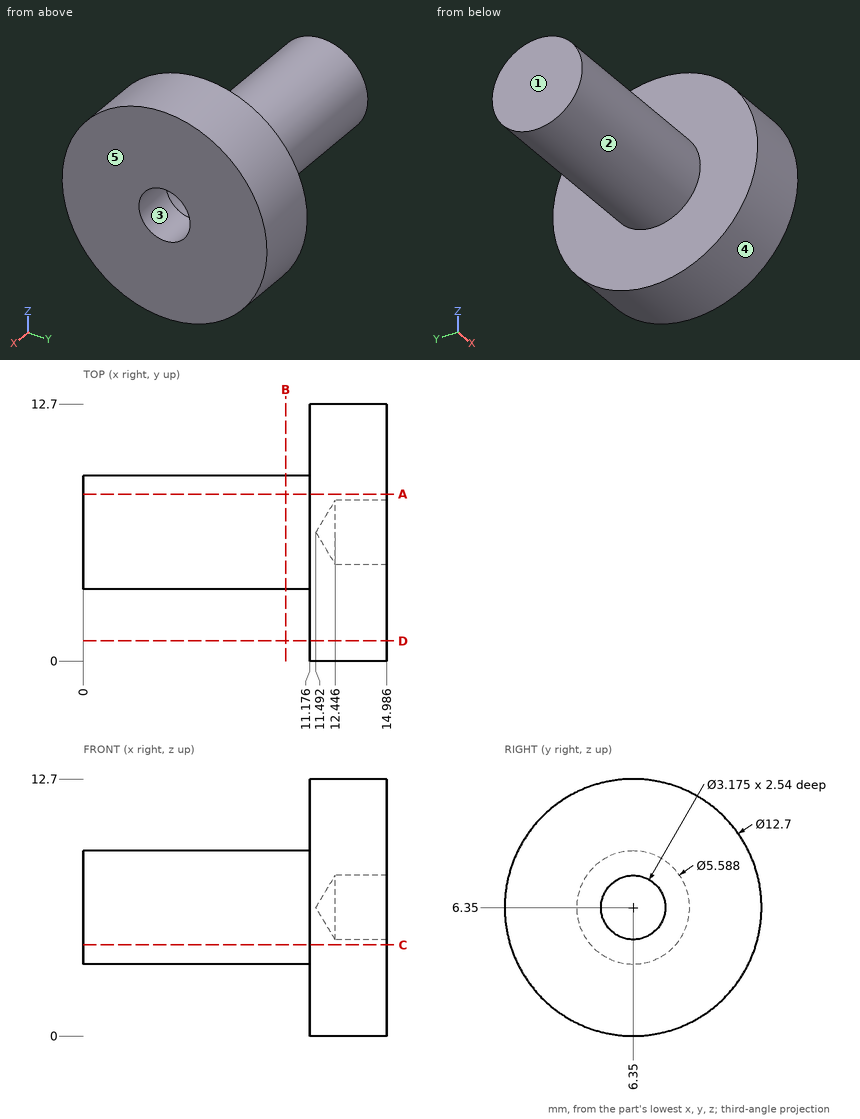
Answer from the drawing. Dimensions are ordinates in mm from the lowest x, y and z of the part. A direction names the side the tool comes from. Give positions to 0.01 mm unless a question says otherwise; leave off trailing zeros. Write each loop counter-clockwise with the first axis right and the second up, starting at its lowest first coordinate (ties: lowest second). Pieces come first, ordered by that corner, then holes.
1) Section C-C (z = 4.5) is taken. Write down the section's boundary in (x, y).
2) A tool of negligible diameter and unlimited length cuts with its end or side. For the marked faces 1 and 2, from which of +Z, -Z, +X, -X, +Y, -Y can it reach the whole face along a straight path? Write none if from no direction.
3) Section D-D (y = 1) is taken. Write down the section's boundary in (x, z), and give its area (3 significant figures).
4) Given P1, Ø6, axis at x = 1.5, y = 11, coming from the -Z side (1 decimal); P2, Ø1, axis at x = 7, z = 4.5, coming from the -Y side; P3, Ø1, axis at x = 4, z = 9, coming from the -Y side (1 decimal), each flat-ended and moving along its own axis, determine where each tip first touches the part or whether it passes through.
5) Find the intervals of material crossed by L1, parallel to Y at x = 14.1, z = 6.35; L2, parallel to X at y = 8.25, z = 10.75; L3, parallel to Z at x = 4.25, y = 6.5, in increasing order.
6) For a pull along Y with two mould halves and no side action, classify the marked faces 3, 4 and 5 as pulls with the +Y half, pulls with the -Y half, needs draft (parallel to the pull), parting line crosses it, or undercut.
7) Section B-B (x = 10) is taken. Write down the section's boundary in (y, z), and give its area (3 significant figures).
8) Section A-A (y = 8.25) is taken. Write down the section's boundary in (x, z).
Response:
1. outline: (0, 4.26) - (11.18, 4.26) - (11.18, 0.28) - (14.99, 0.28) - (14.99, 12.42) - (11.18, 12.42) - (11.18, 8.44) - (0, 8.44) - close
2. face 1: +Z, -Z, -X, +Y, -Y
2. face 2: -X
3. outline: (11.18, 2.93) - (14.99, 2.93) - (14.99, 9.77) - (11.18, 9.77) - close
3. area: 26.1 mm2
4. P1: stops at z = 4.1
4. P2: stops at y = 3.9
4. P3: stops at y = 4.6
5. L1: y = 0 to 4.76, 7.94 to 12.7
5. L2: x = 11.18 to 14.99
5. L3: z = 3.56 to 9.14
6. face 3: undercut
6. face 4: parting line crosses it
6. face 5: needs draft
7. outline: circle Ø5.59 at (6.35, 6.35)
7. area: 24.5 mm2
8. outline: (0, 4.3) - (11.18, 4.3) - (11.18, 0.29) - (14.99, 0.29) - (14.99, 12.41) - (11.18, 12.41) - (11.18, 8.4) - (0, 8.4) - close
